The drawing under review shows one solid part. Ordinate dimensions are in mm from its lowest x, y, z. Round coordinates to 2 decimals unless told otherwise and drop trailing zeros.
1) Mouldability with a two-part tool opening along Y and no side actions: class the marked faces 1, 2 and 3 as pulls with the +Y half, pulls with the -Y half, needs draft (parallel to the pull), parting line crosses it, or undercut.
2) To check wall thickness, follow L1, parallel to Z at x = 10, y = 21.5; L2, parallel to X at y = 9, z = 20 (1 decimal); L3, parallel to X at y = 33, z = 15 (1 decimal). State the ranges of each line that lie inside material, in increasing order.
3) Consider section A-A (y = 10). Give the number of separate pieces and of enclosed holes in the cut face, then the cut area to 3 significant figures.
4) Clearance check with a flat-ended pin moving along its axis: P1, Ø1.2, axis at y = 19.7, z = 27.05, coming from the +X side. State where the tip first meets the part, or that it passes through.
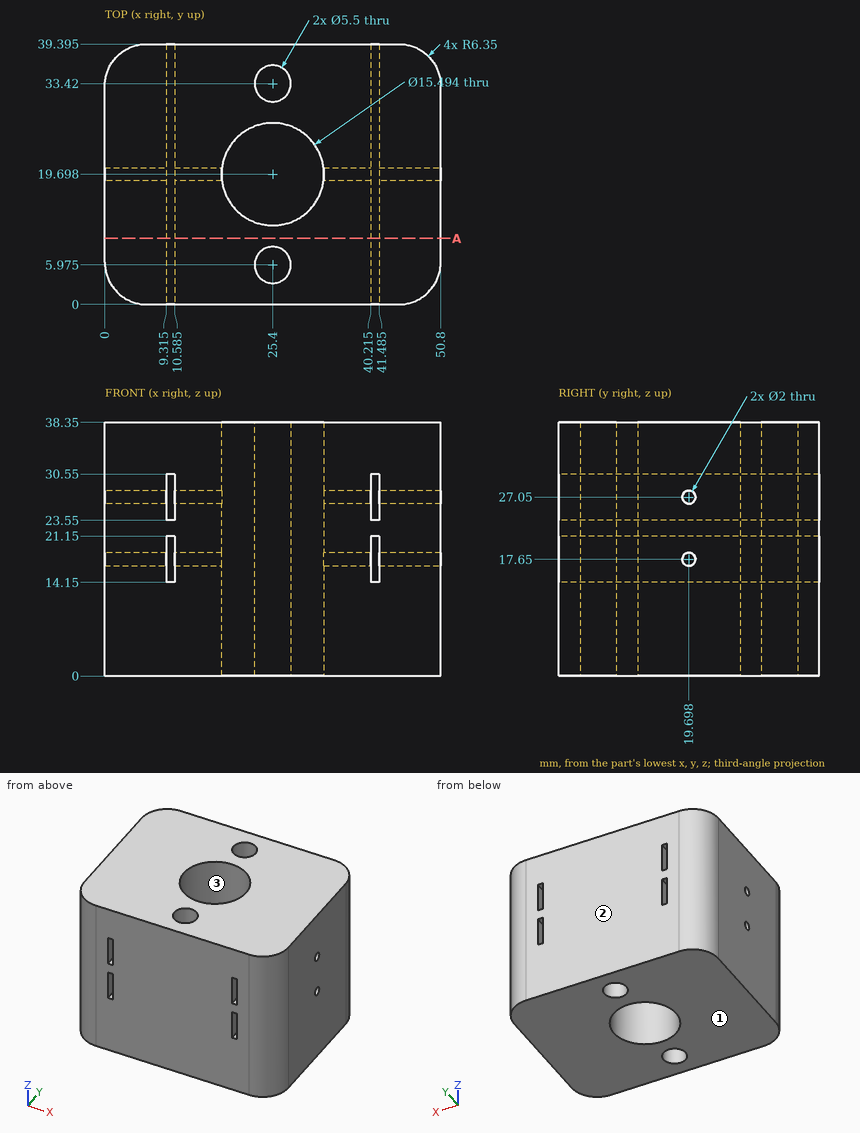
Answer below:
1. face 1: needs draft
1. face 2: pulls with the +Y half
1. face 3: undercut
2. L1: z = 0 to 14.15, 21.15 to 23.55, 30.55 to 38.35
2. L2: x = 0 to 9.3, 10.6 to 40.2, 41.5 to 50.8
2. L3: x = 0 to 9.3, 10.6 to 22.7, 28.1 to 40.2, 41.5 to 50.8
3. separate pieces: 1
3. enclosed holes: 4
3. area: 1,910 mm2
4. P1: passes through
